Could you check a few things on this model? Use its own coordinates, in mm. Face numbers are marked on the shaded views. A direction names the side the tool comes from. Round coordinates to 2 decimals unless told otherwise and drop trailing zeros. Loops run counter-clockwise (first coordinate to the right, second up) from the corner with the lowest first, then second, coordinate; pieces in that order, holes last. Notation, with made-up numbers: M -10,56 L 27,56 A14 cw 27,75 Z; hole C 75.25,36.5 d7. An arc over 180 degrees is marked long. One line per item, written item: value. Start each with the question number.
Q1. Thinking about a two-plate mould opening in X: for the marked faces 3, 4 and 5, which applies, released by +X, released by -X, zero draft, split by the parting line, or undercut?
Q2. I'm going to push flat-ended pins straight in: pin 1 Ø0.6 at (x, z) = (1, 41) entering from +Y; pin 2 Ø4 at (x, y) = (14, 28.5) entering from +Z; pin 3 Ø2 at (x, z) = (45.5, 37) entering from +Y. Where does each tip first touch, or does it pass through?
Q3. Imagine slicing it at D-D (z = 30.5). Please give me the cut outline in (x, y).
Q4. Please list where these lines run through material, in increasing order: line 1 along Y through (x, z) = (13, 13); line 2 along Y through (x, z) = (23.5, 5); line 3 along Y through (x, z) = (33, 35).
Q5. Which directions (+Z, -Z, +X, -X, +Y, -Y) give clear straight access to the entire face, cutting with the end or side of a thin tool? Please do the marked faces 1 and 2.
Q6. Imagine slicing it at A-A (z = 4). Please give me the cut outline in (x, y), then the cut area to 3 significant figures.
Q7. Imagine slicing it at B-B (z = 22). Please give me the cut outline in (x, y), then the cut area to 3 significant figures.
Q8. Imagine slicing it at C-C (y = 46.5). Please give me the cut outline in (x, z).
from build123d import *

# Parameters (mm, degrees)
BOSS_EXTRU_1_DEPTH      = 43
ENL_V_MAT_EXTRU_1_DEPTH = 41
ENL_V_MAT_EXTRU_2_DEPTH = 89.36854644
CHANFREIN1_SIZE         = 1
ENL_V_MAT_EXTRU_3_DEPTH = 89.36854644
ESQUISSE6_W             = 18
ESQUISSE6_H             = 23
BOSS_EXTRU_2_DEPTH      = 18.5
ENL_V_MAT_EXTRU_4_DEPTH = 7
ESQUISSE8_W             = 18
ESQUISSE8_H             = 2
ENL_V_MAT_EXTRU_5_DEPTH = 5.5
ESQUISSE9_W             = 13
ESQUISSE9_H             = 19
ENL_V_MAT_EXTRU_6_DEPTH = 3
CHANFREIN2_SIZE         = 0.5
ENL_V_START             = -11.5
ESQUISSE14_W            = 2.5
ESQUISSE14_H            = 17.5
ENL_V_MAT_EXTRU_7_DEPTH = 11.5
ESQUISSE15_W            = 5.5
ESQUISSE15_H            = 5.5
ESQUISSE15_W_2          = 6
ESQUISSE15_H_2          = 8.5
BOSS_EXTRU_4_DEPTH      = 15
CHANFREIN3_SIZE         = 7
CHANFREIN3_SIZE2        = 4.041451884
CHANFREIN4_SIZE         = 5
CHANFREIN4_SIZE2        = 2.886751346
ESQUISSE16_W            = 10
ESQUISSE16_H            = 8.5
BOSS_EXTRU_5_DEPTH      = 3.11325


with BuildPart() as part:
    # Esquisse1 → Boss.-Extru.1 (new body)
    with BuildSketch(Plane.XY):
        with BuildLine():
            Line((4, 0), (42, 0))
            ThreePointArc((42, 0), (44.828427125, 1.171572875), (46, 4))
            Line((46, 4), (46, 58))
            ThreePointArc((46, 58), (44.828427125, 60.828427125), (42, 62))
            Line((42, 62), (4, 62))
            ThreePointArc((4, 62), (1.171572875, 60.828427125), (0, 58))
            Line((0, 58), (0, 4))
            ThreePointArc((0, 4), (1.171572875, 1.171572875), (4, 0))
        make_face()
    extrude(amount=BOSS_EXTRU_1_DEPTH)

    # Esquisse3 → Enlèv. mat.-Extru.1 (cut)
    with BuildSketch(Plane.XY.offset(43)):
        with BuildLine():
            Line((2, 58), (2, 4))
            ThreePointArc((2, 4), (2.585786438, 2.585786438), (4, 2))
            Line((4, 2), (42, 2))
            ThreePointArc((42, 2), (43.414213562, 2.585786438), (44, 4))
            Line((44, 4), (44, 58))
            ThreePointArc((44, 58), (43.414213562, 59.414213562), (42, 60))
            Line((42, 60), (4, 60))
            ThreePointArc((4, 60), (2.585786438, 59.414213562), (2, 58))
        make_face()
    extrude(amount=-ENL_V_MAT_EXTRU_1_DEPTH, mode=Mode.SUBTRACT)

    # Esquisse4 → Enlèv. mat.-Extru.2 (cut, through all)
    with BuildSketch(Plane(origin=(46, 0, 0), x_dir=(0, 0, -1), z_dir=(1, 0, 0))):
        Polygon((-58.508519511, 60.9), (-39, 60.9), (-39, 58.5), (-33, 58.5), (-33, 54.9), (-39, 54.9), (-39, 52.5), (-58.508519511, 52.5), align=None)
    extrude(amount=-ENL_V_MAT_EXTRU_2_DEPTH, mode=Mode.SUBTRACT)

    # Chanfrein1
    chanfrein1_edges = [part.edges().sort_by_distance(p)[0] for p in [
        (46, 31, 0),
        (44.828427125, 1.171572875, 0),
        (23, 0, 0),
        (1.171572875, 1.171572875, 0),
        (0, 31, 0),
        (1.171572875, 60.828427125, 0),
        (23, 62, 0),
        (44.828427125, 60.828427125, 0),
    ]]
    chamfer(chanfrein1_edges, length=CHANFREIN1_SIZE)

    # Esquisse5 → Enlèv. mat.-Extru.3 (cut, through all)
    with BuildSketch(Plane(origin=(46, 0, 0), x_dir=(0, 0, -1), z_dir=(1, 0, 0))):
        with BuildLine():
            Line((-61.896917985, 37.5), (-15, 37.5))
            ThreePointArc((-15, 37.5), (-13.585786438, 36.914213562), (-13, 35.5))
            Line((-13, 35.5), (-13, 21))
            ThreePointArc((-13, 21), (-13.585786438, 19.585786438), (-15, 19))
            Line((-15, 19), (-61.896917985, 19))
            Line((-61.896917985, 19), (-61.896917985, 37.5))
        make_face()
    extrude(amount=-ENL_V_MAT_EXTRU_3_DEPTH, mode=Mode.SUBTRACT)

    # Esquisse6 → Boss.-Extru.2 (add)
    with BuildSketch(Plane.XY.offset(2)):
        with Locations((21, 35.95)):
            Rectangle(ESQUISSE6_W, ESQUISSE6_H)
    extrude(amount=BOSS_EXTRU_2_DEPTH)

    # Esquisse7 → Enlèv. mat.-Extru.4 (cut)
    with BuildSketch(Plane.XY.offset(20.5)):
        Polygon((12, 41.95), (12, 47.45), (30, 47.45), (30, 41.95), (27.25, 41.95), (27.25, 24.45), (14.75, 24.45), (14.75, 41.95), align=None)
    extrude(amount=-ENL_V_MAT_EXTRU_4_DEPTH, mode=Mode.SUBTRACT)

    # Esquisse8 → Enlèv. mat.-Extru.5 (cut)
    with BuildSketch(Plane.XY.offset(13.5)):
        with Locations((21, 42.95)):
            Rectangle(ESQUISSE8_W, ESQUISSE8_H)
    extrude(amount=-ENL_V_MAT_EXTRU_5_DEPTH, mode=Mode.SUBTRACT)

    # Esquisse9 → Enlèv. mat.-Extru.6 (cut)
    with BuildSketch(Plane.XZ):
        with Locations((23.5, 33.5)):
            Rectangle(ESQUISSE9_W, ESQUISSE9_H)
    extrude(amount=-ENL_V_MAT_EXTRU_6_DEPTH, mode=Mode.SUBTRACT)

    # Chanfrein2
    chanfrein2_edges = [part.edges().sort_by_distance(p)[0] for p in [
        (21, 43.95, 13.5),
    ]]
    chamfer(chanfrein2_edges, length=CHANFREIN2_SIZE)

    # Esquisse14 → Enlèv. mat.-Extru.7 (cut)
    with BuildSketch(Plane.XY.offset(13.5).offset(ENL_V_START)):
        with Locations((21, 33.2)):
            Rectangle(ESQUISSE14_W, ESQUISSE14_H)
    extrude(amount=ENL_V_MAT_EXTRU_7_DEPTH, mode=Mode.SUBTRACT)

    # Esquisse15 → Boss.-Extru.4 (add)
    with BuildSketch(Plane.XY.offset(2)):
        with Locations((4.75, 57.25)):
            Rectangle(ESQUISSE15_W, ESQUISSE15_H)
        with Locations((41, 55.75)):
            Rectangle(ESQUISSE15_W_2, ESQUISSE15_H_2)
    extrude(amount=BOSS_EXTRU_4_DEPTH)

    # Chanfrein3
    chanfrein3_edges = [part.edges().sort_by_distance(p)[0] for p in [
        (7.5, 57.25, 17),
    ]]
    chanfrein3_side = [part.faces().sort_by_distance(p)[0] for p in [
        (7.5, 57.25, 9.5),
    ]]
    chamfer(chanfrein3_edges, length=CHANFREIN3_SIZE, length2=CHANFREIN3_SIZE2, reference=chanfrein3_side[0])

    # Chanfrein4
    chanfrein4_edges = [part.edges().sort_by_distance(p)[0] for p in [
        (38, 55.75, 17),
    ]]
    chanfrein4_side = [part.faces().sort_by_distance(p)[0] for p in [
        (38, 55.75, 9.5),
    ]]
    chamfer(chanfrein4_edges, length=CHANFREIN4_SIZE, length2=CHANFREIN4_SIZE2, reference=chanfrein4_side[0])

    # Esquisse16 → Boss.-Extru.5 (add)
    with BuildSketch(Plane.ZY.offset(-44)):
        with Locations((22, 55.75)):
            Rectangle(ESQUISSE16_W, ESQUISSE16_H)
    extrude(amount=BOSS_EXTRU_5_DEPTH)


solid = part.part
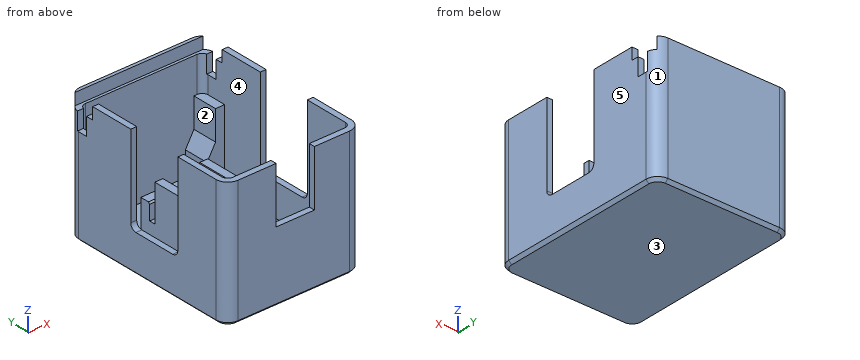
Report:
1. face 3: zero draft
1. face 4: undercut
1. face 5: released by +X
2. pin 1: stops at y = 60.95
2. pin 2: stops at z = 20.5
2. pin 3: stops at y = 61.12
3. outline: M 0,4 A4 ccw 4,0 L 17,0 L 17,2 L 4,2 A2 cw 2,4 L 2,19 L 0,19 Z; M 0,37.5 L 2,37.5 L 2,58 A2 cw 4,60 L 42,60 A2 cw 44,58 L 44,37.5 L 46,37.5 L 46,58 A4 ccw 42,62 L 4,62 A4 ccw 0,58 Z; M 30,0 L 42,0 A4 ccw 46,4 L 46,19 L 44,19 L 44,4 A2 cw 42,2 L 30,2 Z
4. line 1: y = 0 to 2, 24.45 to 41.95, 43.95 to 47.45, 60 to 62
4. line 2: y = 0 to 2, 24.45 to 47.45, 60 to 62
4. line 3: y = 0 to 2, 60 to 62
5. face 1: +Z, -Z, +X, +Y
5. face 2: +Z
6. outline: M 0,4 A4 ccw 4,0 L 42,0 A4 ccw 46,4 L 46,58 A4 ccw 42,62 L 4,62 A4 ccw 0,58 Z; M 12,24.45 L 19.75,24.45 L 19.75,41.95 L 22.25,41.95 L 22.25,24.45 L 30,24.45 L 30,47.45 L 12,47.45 Z; hole M 2,4 A2 ccw 4,2 L 42,2 A2 ccw 44,4 L 44,51.5 L 38,51.5 L 38,60 L 7.5,60 L 7.5,54.5 L 2,54.5 Z
6. area: 855 mm²
7. outline: M 0,4 A4 ccw 4,0 L 42,0 A4 ccw 46,4 L 46,19 L 44,19 L 44,4 A2 cw 42,2 L 4,2 A2 cw 2,4 L 2,19 L 0,19 Z; M 0,37.5 L 2,37.5 L 2,58 A2 cw 4,60 L 40.89,60 L 40.89,51.5 L 44,51.5 L 44,37.5 L 46,37.5 L 46,58 A4 ccw 42,62 L 4,62 A4 ccw 0,58 Z
7. area: 357 mm²
8. outline: M 0,1 L 1,0 L 45,0 L 46,1 L 46,43 L 44,43 L 44,2 L 30,2 L 30,13.5 L 12,13.5 L 12,2 L 2,2 L 2,43 L 0,43 Z
